Part model, mm, in its own coordinate system. Face numbers are marked on the shaded views. Round coordinates to 2 decimals unless told otherwise and drop trailing zeros. Write each loop counter-clockwise with the first axis right and the second up, starting at its lowest first coordinate (ties: lowest second). Pieces come first, ordered by that corner, then holes. Notation, with made-up numbers: (71, 33.5) -> (99, 33.5) arc R24 ccw to (99, 49.5) -> close; hole circle Ø4 at (17, 39). An arc over 180 degrees is marked (long way). Use CSV: the item, a comma, the result in double quotes. Start each with the question number.
(1) Saw through at A-A (x = 97.5). Give the cut face in (y, z).
(2) Saw through at D-D (y = 440.5). Give the cut face in (x, z), plus the area to 3 significant figures.
(3) Two-plate mould, pull along Y, no slides. Class the marked faces 1, 2 and 3: released by +Y, released by -Y, zero draft, split by the parting line, or undercut.
(4) Probe line 1 (X direction, y = 419.5, z = 21.7); line 2 (Y direction, x = 86.5, z = 19.4); line 3 (Y direction, x = 89.5, z = 20.3). List the from-to ranges inside material, lowest first. Write a range as [from, to].
(5) Saw through at C-C (z = 22.95). Count the separate pieces of the cut face and the enclosed holes in it, plus the area to 3 significant figures.
(6) Drop flat-ended pins along their axis: pin 1 (6 mm diameter, centred on x = 93.5, y = 445, fed in from -Z); pin 2 (1 mm diameter, centred on x = 101, z = 19.5, fed in from -Y); pin 3 (1 mm diameter, centred on x = 44.5, z = 20, fed in from -Y). Give the stop position or say it passes through.
(7) Saw through at B-B (x = 70). Give the cut face in (y, z).
```python
from build123d import *

# Parameters (mm, degrees)
SKETCH_W            = 61.775986
SKETCH_H            = 42.418
PAD_DEPTH           = 2
PAD_DEPTH_BACK      = 4
SKETCH001_R         = 1.7
HOLE_DEPTH          = 25
HOLE001_D           = 3.4
HOLE001_DEPTH       = 25
HOLE001_CBORE_D     = 6
HOLE001_CBORE_DEPTH = 2.4
FILLET_R            = 5
SKETCH003_W         = 25.4
SKETCH003_H         = 4.354827
POCKET_DEPTH        = 61.776986


with BuildPart() as part:
    # Sketch (on Face4 of Binder) → Pad (new body, two sides)
    with BuildSketch(Plane(origin=(0, 0, 20.8), x_dir=(1, 0, 0), z_dir=(0, 0, -1))) as pad_sk:
        with Locations((72.221347, -434.991848)):
            Rectangle(SKETCH_W, SKETCH_H)
    extrude(amount=PAD_DEPTH)
    extrude(pad_sk.sketch, amount=-PAD_DEPTH_BACK)

    # Sketch001 (on Face5 of Pad) → Hole (cut)
    with BuildSketch(Plane.XY.offset(24.8)):
        with Locations((87.721347, 450.491848)):
            Circle(SKETCH001_R)
        with Locations((56.721347, 450.491848)):
            Circle(SKETCH001_R)
        with Locations((87.721347, 419.491848)):
            Circle(SKETCH001_R)
        with Locations((56.721347, 419.491848)):
            Circle(SKETCH001_R)
        with Locations((46.721347, 419.491848)):
            Circle(SKETCH001_R)
        with Locations((46.721347, 450.491848)):
            Circle(SKETCH001_R)
        with Locations((97.721347, 419.491848)):
            Circle(SKETCH001_R)
        with Locations((97.721347, 450.491848)):
            Circle(SKETCH001_R)
    extrude(amount=-HOLE_DEPTH, mode=Mode.SUBTRACT)

    # Hole001
    with Locations(Plane(origin=(0, 0, 18.8), x_dir=(1, 0, 0), z_dir=(0, 0, -1))):
        with Locations((56.721347, -419.491848), (87.721347, -419.491848), (87.721347, -450.491848), (56.721347, -450.491848)):
            CounterBoreHole(HOLE001_D / 2, HOLE001_CBORE_D / 2, HOLE001_CBORE_DEPTH, depth=HOLE001_DEPTH)

    # Fillet
    fillet_edges = [part.edges().sort_by_distance(p)[0] for p in [
        (41.333354, 413.782848, 21.8),
        (103.10934, 413.782848, 21.8),
        (103.10934, 456.200848, 21.8),
        (41.333354, 456.200848, 21.8),
    ]]
    fillet(fillet_edges, radius=FILLET_R)

    # Sketch003 (on Face7 of Fillet) → Pocket (cut, through all)
    with BuildSketch(Plane.YZ.offset(103.10934)):
        with Locations((436.5, 18.622587)):
            Rectangle(SKETCH003_W, SKETCH003_H)
    extrude(amount=-POCKET_DEPTH, mode=Mode.SUBTRACT)


solid = part.part
```
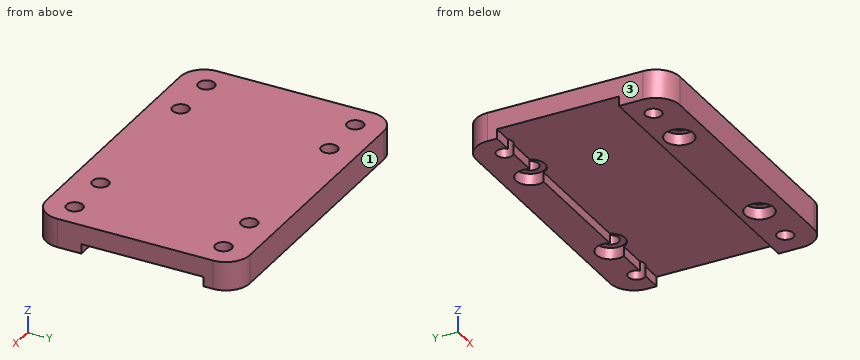
Answers:
1,outline,"(413.78, 18.8) -> (417.81, 18.8) -> (417.81, 24.8) -> (413.78, 24.8) -> close; (421.18, 18.8) -> (423.8, 18.8) -> (423.8, 20.8) -> (448.81, 20.8) -> (448.81, 24.8) -> (421.18, 24.8) -> close; (452.18, 18.8) -> (456.2, 18.8) -> (456.2, 24.8) -> (452.18, 24.8) -> close"
2,outline,"(41.33, 20.8) -> (103.11, 20.8) -> (103.11, 24.8) -> (41.33, 24.8) -> close"
2,area,"247 mm²"
3,face 1,"released by +Y"
3,face 2,"undercut"
3,face 3,"zero draft"
4,line 1,"x = [41.33, 45.02], [48.42, 55.02], [58.42, 86.02], [89.42, 96.02], [99.42, 103.11]"
4,line 2,"y = [413.78, 416.75], [422.23, 423.8], [453.23, 456.2]"
4,line 3,"y = [413.78, 417.08], [421.91, 423.8], [452.91, 456.2]"
5,separate pieces,"1"
5,enclosed holes,"8"
5,area,"2,530 mm²"
6,pin 1,"stops at z = 20.8"
6,pin 2,"stops at y = 414.39"
6,pin 3,"stops at y = 413.96"
7,outline,"(413.78, 18.8) -> (423.8, 18.8) -> (423.8, 20.8) -> (449.2, 20.8) -> (449.2, 18.8) -> (456.2, 18.8) -> (456.2, 24.8) -> (413.78, 24.8) -> close"
